```python
from build123d import *

# Parameters (mm, degrees)
F0_R     = 15
F1_DEPTH = 12.5
F3_DEPTH = 5
F4_R     = 4.25
F5_DEPTH = 20.001
F6_R     = 5
F7_SIZE  = 1
F8_R     = 1.5
F9_DEPTH = 50


with BuildPart() as f1:
    # F0 (on Top) → F1 (new body, symmetric)
    with BuildSketch(Plane.XY):
        Circle(F0_R)
    extrude(amount=F1_DEPTH, both=True)

    # F2 (on face) → F3 (cut)
    with BuildSketch(Plane.XY.offset(12.5)):
        Polygon((6.5, -3.752777), (6.5, 3.752777), (0, 7.505553), (-6.5, 3.752777), (-6.5, -3.752777), (0, -7.505553), align=None)
    extrude(amount=-F3_DEPTH, mode=Mode.SUBTRACT)

    # F4 (on face) → F5 (cut, through all)
    with BuildSketch(Plane.XY.offset(7.5)):
        Circle(F4_R)
    extrude(amount=-F5_DEPTH, mode=Mode.SUBTRACT)

    # F6
    f6_edges = [f1.edges().sort_by_distance(p)[0] for p in [
        (-15, 0, 12.5),
        (-15, 0, -12.5),
    ]]
    fillet(f6_edges, radius=F6_R)

    # F7
    f7_edges = [f1.edges().sort_by_distance(p)[0] for p in [
        (-4.25, 0, -12.5),
    ]]
    chamfer(f7_edges, length=F7_SIZE)

    # F8 (on Front) → F9 (cut)
    with BuildSketch(Plane.XZ):
        Circle(F8_R)
    extrude(amount=-F9_DEPTH, mode=Mode.SUBTRACT)


solid = f1.part
```
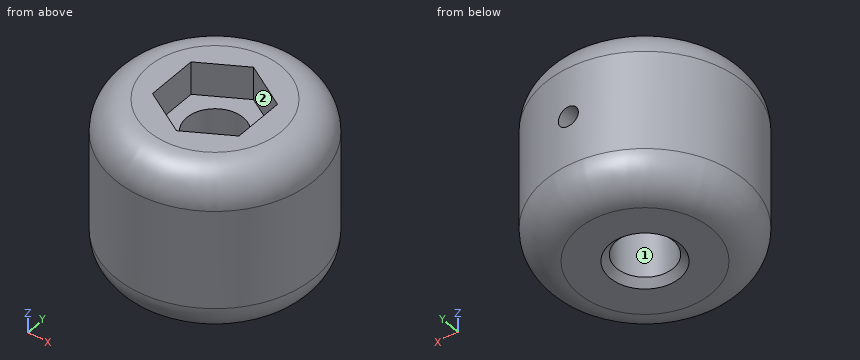
Here's how the part is built. I have some questions about the finished solid (model axes, mm). Face numbers are marked on the shaded views. A direction names the side the tool comes from. Coordinates: 2 decimals unless noted, no trailing zeros. Order: outer loops, then holes, each group sorted by start corner. A loop starts at its lowest first (then second) coordinate and runs counter-clockwise, first axis right, second up.
1) Imagine slicing it at D-D on z = 0. List the corners of the cut face in (x, y) for me, and give its area (3 significant figures).
2) Will these pins go through, and if not, where does the flat tip stop? pin 1 (6 mm diameter, centred on y = -11.5, z = -4, fed in from -X); pin 2 (8 mm diameter, centred on y = -6.5, z = 9, fed in from +X); pin 3 (1 mm diameter, centred on y = 7.5, z = 2.5, fed in from +X).
3) Which directions (+Z, -Z, +X, -X, +Y, -Y) give clear straight access to the entire face, cutting with the end or side of a thin tool? Please do the marked faces 1 and 2.
4) Imagine slicing it at A-A on y = 0. List the corners of the cut face in (x, z) for me, and give its area (3 significant figures).
5) I need wall thicknesses on line 1 (Z direction, x = 0, y = 9.5); line 2 (X direction, y = 3, z = 7.25); line 3 (Y direction, x = 6, z = 10.25). Which ranges of each line are inside material? Lowest first, please.
6) Imagine slicing it at C-C on x = 0.5. State how many separate pieces and enclosed holes the cut face has, and give its area (3 significant figures).
7) Imagine slicing it at B-B on z = 9.5. List the corners of the cut face in (x, y) for me.
Response values:
1. outline: (-1.5, 3.98) - (-1.5, 14.92) arc R15 ccw (long way) to (1.5, 14.92) - (1.5, 3.98) arc R4.25 cw (long way) to start
1. area: 618 mm2
2. pin 1: stops at x = -12.36
2. pin 2: stops at x = 14.75
2. pin 3: stops at x = 13.27
3. face 1: +Z, -Z
3. face 2: +Z
4. outline: (-15, -7.5) arc R5 ccw to (-10, -12.5) - (-5.25, -12.5) - (-4.25, -11.5) - (-4.25, 7.5) - (-6.5, 7.5) - (-6.5, 12.5) - (-10, 12.5) arc R5 ccw to (-15, 7.5) - close; (4.25, -11.5) - (5.25, -12.5) - (10, -12.5) arc R5 ccw to (15, -7.5) - (15, 7.5) arc R5 ccw to (10, 12.5) - (6.5, 12.5) - (6.5, 7.5) - (4.25, 7.5) - close
4. area: 493 mm2
5. line 1: z = -12.5 to -1.5, 1.5 to 12.5
5. line 2: x = -14.7 to -3.01, 3.01 to 14.7
5. line 3: y = -12.84 to -4.04, 4.04 to 12.84
6. separate pieces: 3
6. enclosed holes: 0
6. area: 456 mm2
7. outline: circle Ø29.17 at (0, 0); hole (-6.5, -3.75) - (0, -7.51) - (6.5, -3.75) - (6.5, 3.75) - (0, 7.51) - (-6.5, 3.75) - close
